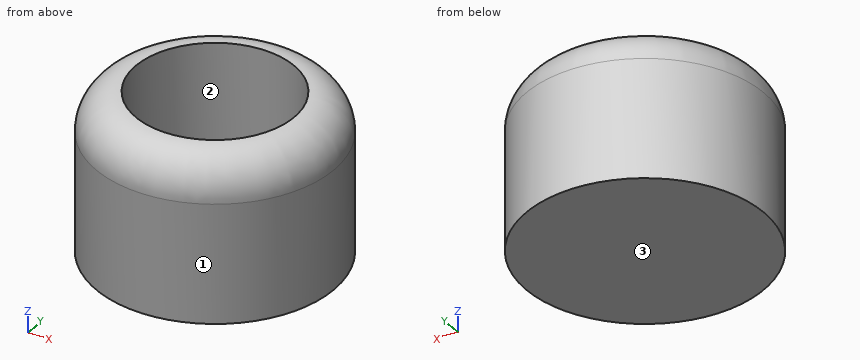
from build123d import *

# Parameters (mm, degrees)
F0_W = 76.2
F0_H = 101.6
F2_R = 25.4
F3_T = -25.4


# Not quite as in the source:
# - a shell that OpenCascade refuses in one call is made with other operations: the cavity is built on its own and cut out


with BuildPart() as f1:
    # F0 (on Front) → F1 (revolve)
    with BuildSketch(Plane.XZ):
        with Locations((-38.1, 0)):
            Rectangle(F0_W, F0_H)
    revolve(axis=Axis((0, 0, 0), (0, 0, -1)))

    # F2
    f2_edges = [f1.edges().sort_by_distance(p)[0] for p in [
        (76.2, 0, 50.8),
    ]]
    fillet(f2_edges, radius=F2_R)

    # F3: a shell. OpenCascade refuses it in one call, so the cavity is built on its own and cut out:
    # the body offset inwards by the wall thickness, plus a prism from it out through each open face.
    f3_core = offset(f1.part, amount=F3_T, kind=Kind.INTERSECTION, mode=Mode.PRIVATE)
    f3_exits = [f3_core.faces().sort_by_distance(p)[0] for p in [
        (0, 0, 25.4),
    ]]
    add(f3_core, mode=Mode.SUBTRACT)
    extrude(f3_exits, amount=-F3_T, mode=Mode.SUBTRACT)


solid = f1.part
The listing builds one solid part. Answer for the finished solid, in the listing's coordinates (mm). Face numbers are marked on the shaded views. Coordinates: 2 decimals unless noted, no trailing zeros. Order: outer loops, then holes, each group sorted by start corner. A loop starts at its lowest first (then second) coordinate and runs counter-clockwise, first axis right, second up. Notation, with made-up numbers: (55.5, 60.25) -> (108.5, 60.25) arc R28 cw to (108.5, 90.25) -> close; hole circle Ø10 at (48.25, 4). An arc over 180 degrees is marked (long way). Answer in a Markdown table with one row per item. Add a question column.
Item 1: Each of these flat-tipped pins is pushed along its axis until it touches: P1, Ø5, axis at x = 13, z = -30, coming from the -Y side; P2, Ø3, axis at x = 37.5, z = 13, coming from the +Y side; P3, Ø1.5, axis at y = 13, z = 1, coming from the +X side. Where does it stop, or does it pass through?
Item 2: Find section C-C (z = 17). Write down the section's boundary in (x, y), then the cut area to 3 significant figures.
Item 3: Find section A-A (x = 0). Write down the section's boundary in (y, z), then the cut area to 4 significant figures.
Item 4: Determine the mould class of the marked faces 1, 2 and 3 for opening direction Y: +Y half, -Y half, draft (parallel to the pull), parting line (faces both ways), or undercut.
Item 5: Find section D-D (z = 35.5). Write down the section's boundary in (x, y).
Item 6: Find the intervals of material crossed by L1, parallel to Y at x = 0, z = 13; L2, parallel to X at y = 17.5, z = -1; L3, parallel to Y at x = -19.5, z = -9.5, in increasing order. Write a range as from..to.
Result set:
| question | item | result |
|---|---|---|
| 1 | P1 | stops at y = -75.47 |
| 1 | P2 | stops at y = 67.16 |
| 1 | P3 | stops at x = 75.21 |
| 2 | outline | circle Ø152.4 at (0, 0); hole circle Ø101.6 at (0, 0) |
| 2 | area | 10,100 mm² |
| 3 | outline | (-76.2, -50.8) -> (76.2, -50.8) -> (76.2, 25.4) arc R25.4 ccw to (50.8, 50.8) -> (50.8, -25.4) -> (-50.8, -25.4) -> (-50.8, 50.8) arc R25.4 ccw to (-76.2, 25.4) -> close |
| 3 | area | 7,465 mm² |
| 4 | face 1 | parting line |
| 4 | face 2 | undercut |
| 4 | face 3 | draft |
| 5 | outline | circle Ø148.21 at (0, 0); hole circle Ø101.6 at (0, 0) |
| 6 | L1 | y = -76.2..-50.8, 50.8..76.2 |
| 6 | L2 | x = -74.16..-47.69, 47.69..74.16 |
| 6 | L3 | y = -73.66..-46.91, 46.91..73.66 |
